from build123d import *

# Parameters (mm, degrees)
SKETCH1_R           = 13.35
SKETCH1_R_2         = 12.6
SKETCH1_R_3         = 1.575
BOSS_EXTRUDE1_DEPTH = 1
SKETCH1_3_R         = 12.6
SKETCH1_3_R_2       = 1.575
BOSS_EXTRUDE2_DEPTH = 6
SKETCH2_R           = 3
CUT_EXTRUDE1_DEPTH  = 3.5


with BuildPart() as part:
    # Sketch1 → Boss-Extrude1 (new body)
    # profile 1 of 2: a face of its own
    with BuildSketch(Plane(origin=(0, 33, 0), x_dir=(1, 0, 0), z_dir=(0, 1, 0))):
        with Locations(Location((0, 0, 0), (0, 0, 270))):
            Circle(SKETCH1_R)
        Circle(SKETCH1_R_2, mode=Mode.SUBTRACT)
    # profile 2 of 2: a face of its own
    with BuildSketch(Plane(origin=(0, 33, 0), x_dir=(1, 0, 0), z_dir=(0, 1, 0))):
        Circle(SKETCH1_R_2)
        with Locations(Location((6, -6, 0), (0, 0, 270))):
            Circle(SKETCH1_R_3, mode=Mode.SUBTRACT)
        with Locations(Location((-6, 6, 0), (0, 0, 270))):
            Circle(SKETCH1_R_3, mode=Mode.SUBTRACT)
        with Locations(Location((6, 6, 0), (0, 0, 270))):
            Circle(SKETCH1_R_3, mode=Mode.SUBTRACT)
        with Locations(Location((-6, -6, 0), (0, 0, 270))):
            Circle(SKETCH1_R_3, mode=Mode.SUBTRACT)
    extrude(amount=BOSS_EXTRUDE1_DEPTH)

    # Sketch1<3> → Boss-Extrude2 (add)
    with BuildSketch(Plane(origin=(0, 33, 0), x_dir=(1, 0, 0), z_dir=(0, 1, 0))):
        with Locations(Location((0, 0, 0), (0, 0, 270))):
            Circle(SKETCH1_3_R)
        with Locations(Location((6, -6, 0), (0, 0, 270))):
            Circle(SKETCH1_3_R_2, mode=Mode.SUBTRACT)
        with Locations(Location((-6, 6, 0), (0, 0, 270))):
            Circle(SKETCH1_3_R_2, mode=Mode.SUBTRACT)
        with Locations(Location((6, 6, 0), (0, 0, 270))):
            Circle(SKETCH1_3_R_2, mode=Mode.SUBTRACT)
        with Locations(Location((-6, -6, 0), (0, 0, 270))):
            Circle(SKETCH1_3_R_2, mode=Mode.SUBTRACT)
    extrude(amount=BOSS_EXTRUDE2_DEPTH)

    # Sketch2 → Cut-Extrude1 (cut)
    with BuildSketch(Plane(origin=(0, 39, 0), x_dir=(1, 0, 0), z_dir=(0, 1, 0))):
        with Locations(Location((-6, 6, 0), (0, 0, 270))):
            Circle(SKETCH2_R)
        with Locations(Location((6, 6, 0), (0, 0, 270))):
            Circle(SKETCH2_R)
        with Locations(Location((6, -6, 0), (0, 0, 270))):
            Circle(SKETCH2_R)
        with Locations(Location((-6, -6, 0), (0, 0, 270))):
            Circle(SKETCH2_R)
    extrude(amount=-CUT_EXTRUDE1_DEPTH, mode=Mode.SUBTRACT)


solid = part.part
For this review, take the finished solid that the model builds, in its own axes (mm). A direction names the side the tool comes from. Give positions to 0.01 mm unless a question says otherwise; leave off trailing zeros. Loops run counter-clockwise (first coordinate to the right, second up) from the corner with the lowest first, then second, coordinate; pieces in that order, holes last. Notation, with made-up numbers: (32.5, 81) - (52.5, 81) arc R18 cw to (52.5, 93) - close; hole circle Ø8 at (19, 39). An arc over 180 degrees is marked (long way). Write each question's results on one line, items separated by ' | '.
(1) Take a section at B-B (y = 34.5). Give the boundary of the cut face in (x, z) (3 decimals), then the cut area to 3 significant figures.
Conclusion:
outline: circle Ø25.2 at (0, 0); hole circle Ø3.15 at (-6, -6); hole circle Ø3.15 at (-6, 6); hole circle Ø3.15 at (6, -6); hole circle Ø3.15 at (6, 6) | area: 468 mm^2
(2) Take a section at D-D (x = 0). Give the boundary of the cut face in (y, z), then the cut area to 3 significant figures.
Conclusion:
outline: (33, -13.35) - (34, -13.35) - (34, -12.6) - (39, -12.6) - (39, 12.6) - (34, 12.6) - (34, 13.35) - (33, 13.35) - close | area: 153 mm^2
(3) For line 1 along Z through (x, y) = (6, 34.95) (3 decimals); line 2 along X through (y, z) = (36.35, -6), list the stretches that pass through material, from the lowest coordinate up.
Conclusion:
line 1: -11.08 to -7.575, -4.425 to 4.425, 7.575 to 11.08 | line 2: -11.08 to -9, -3 to 3, 9 to 11.08
(4) Take a section at C-C (x = 4.75). Give the boundary of the cut face in (y, z).
Conclusion:
outline: (33, -12.48) - (34, -12.48) - (34, -11.67) - (39, -11.67) - (39, -8.73) - (35.5, -8.73) - (35.5, -6.96) - (33, -6.96) - close; (33, -5.04) - (35.5, -5.04) - (35.5, -3.27) - (39, -3.27) - (39, 3.27) - (35.5, 3.27) - (35.5, 5.04) - (33, 5.04) - close; (33, 6.96) - (35.5, 6.96) - (35.5, 8.73) - (39, 8.73) - (39, 11.67) - (34, 11.67) - (34, 12.48) - (33, 12.48) - close
(5) For faces 4 (the cylindrical face through (-7.667, 36.465, -9.999)), 5 (the flat face through (0, 39, 0)), list the 3-axis set-ups (+Z, -Z, +X, -X, +Y, -Y) from which the entire face can be reached by the end or side of a thin tool; tool diameter is ignored.
Conclusion:
face 4: +Y | face 5: +Z, -Z, +X, -X, +Y
(6) Take a section at A-A (z = -6). Give the boundary of the cut face in (x, y) (3 decimals).
Conclusion:
outline: (-11.926, 33) - (-7.575, 33) - (-7.575, 35.5) - (-9, 35.5) - (-9, 39) - (-11.08, 39) - (-11.08, 34) - (-11.926, 34) - close; (-4.425, 33) - (4.425, 33) - (4.425, 35.5) - (3, 35.5) - (3, 39) - (-3, 39) - (-3, 35.5) - (-4.425, 35.5) - close; (7.575, 33) - (11.926, 33) - (11.926, 34) - (11.08, 34) - (11.08, 39) - (9, 39) - (9, 35.5) - (7.575, 35.5) - close
(7) Draft analysis for pull direction Z (two halves, no side actions). For faces 1 (the flat face through (0, 33, 0)), 2 (the cylindrical face through (-5.113, 33.493, 12.332)), 3 (the cylindrical face through (3.338, 37.274, -4.616)), state which applies: +Z half, -Z half, draft (parallel to the pull), parting line (faces both ways), or undercut.
Conclusion:
face 1: draft | face 2: parting line | face 3: undercut
(8) For pin 1 Ø3 at (y, z) = (38.5, 5.5) entering from +X; pin 2 Ø5 at (x, z) = (6, -6) entering from +Y; pin 3 Ø4 at (x, z) = (-6, 6) entering from -Y; pin 4 Ø1.8 at (x, z) = (5.5, -6) entering from +Y, all flat-tipped, find the tip position at first contact; note any pin that passes through.
Conclusion:
pin 1: x = 11.95 | pin 2: y = 35.5 | pin 3: y = 33 | pin 4: through
